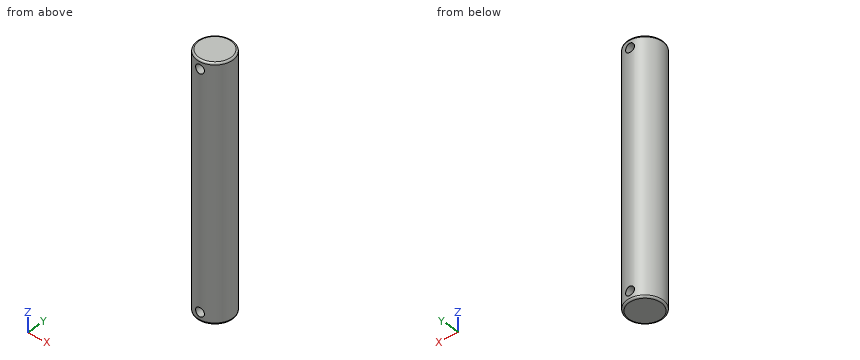
from build123d import *

# Parameters (mm, degrees)
SKETCH1_R               = 10
BOSS_EXTRUDE1_DEPTH     = 140
FILLET1_R               = 1
CUT_EXTRUDE1_DEPTH      = 140
CUT_EXTRUDE1_DEPTH_BACK = 140
SKETCH2_R               = 2.5


with BuildPart() as part:
    # Sketch1 → Boss-Extrude1 (new body)
    with BuildSketch(Plane.XY):
        Circle(SKETCH1_R)
    extrude(amount=BOSS_EXTRUDE1_DEPTH)

    # Fillet1
    fillet1_edges = [part.edges().sort_by_distance(p)[0] for p in [
        (-10, 0, 0),
        (-10, 0, 140),
    ]]
    fillet(fillet1_edges, radius=FILLET1_R)

    # Sketch2 → Cut-Extrude1 (cut, two sides: drawn at the far end of the back side and taken through both)
    with BuildSketch(Plane(origin=(0, 0, 0), x_dir=(1, 0, 0), z_dir=(0, 1, 0)).offset(-CUT_EXTRUDE1_DEPTH_BACK)):
        with Locations(Location((0, -5, 0), (0, 0, 90))):
            Circle(SKETCH2_R)
        with Locations(Location((0, -135, 0), (0, 0, 90))):
            Circle(SKETCH2_R)
    extrude(amount=CUT_EXTRUDE1_DEPTH + CUT_EXTRUDE1_DEPTH_BACK, mode=Mode.SUBTRACT)


solid = part.part
Design review of the part built by this model. Coordinates are the model's own, in mm. Coordinates: 2 decimals unless noted, no trailing zeros. Write each loop counter-clockwise with the first axis right and the second up, starting at its lowest first coordinate (ties: lowest second). Pieces come first, ordered by that corner, then holes. Notation, with made-up numbers: (-33.5, 48) -> (-23.5, 48) arc R17 ccw to (-23.5, 72) -> close; hole circle Ø10 at (-14.75, 25). An arc over 180 degrees is marked (long way). Write each question's results on one line, items separated by ' | '. Start each with the question number.
(1) Take a section at A-A on x = 0. Write out the cut boundary in (y, z), and give its area (3 significant figures).
(2) Take a section at B-B on z = 58. Write out the cut boundary in (x, y).
(3) Take a section at C-C on y = 3.25. Give the number of separate pieces and of enclosed holes in the cut face, and give its area (3 significant figures).
(4) Clearance check with flat-ended pins moving along their axes: P1, Ø1.5, axis at x = 8, z = 107.5, coming from the -Y side; P2, Ø4.5, axis at x = 0, z = 5, coming from the -Y side; P3, Ø6, axis at x = 7.5, z = 84.5, coming from the +Y side. State where each tip first meets the part, or that it passes through.
(5) Take a section at D-D on z = 5. Write out the cut boundary in (x, y).
(6) For line 1 along Z through (x, y) = (-1.75, -3.25); line 2 along Z through (x, y) = (0.5, -7); line 3 along X through (y, z) = (3.5, 5), list the stretches that pass through material, from the lowest coordinate up. Write a range as from..to.
Results found:
1) outline: (-10, 1) arc R1 ccw to (-9, 0) -> (9, 0) arc R1 ccw to (10, 1) -> (10, 2.5) -> (-10, 2.5) -> close; (-10, 7.5) -> (10, 7.5) -> (10, 132.5) -> (-10, 132.5) -> close; (-10, 137.5) -> (10, 137.5) -> (10, 139) arc R1 ccw to (9, 140) -> (-9, 140) arc R1 ccw to (-10, 139) -> close | area: 2,600 mm2
2) outline: circle Ø20 at (0, 0)
3) separate pieces: 1 | enclosed holes: 2 | area: 2,610 mm2
4) P1: stops at y = -6.89 | P2: passes through | P3: stops at y = 8.93
5) outline: (-2.5, -9.68) -> (-2.5, 9.68) arc R10 ccw to start; (2.5, -9.68) arc R10 ccw to (2.5, 9.68) -> close
6) line 1: z = 0..3.21, 6.79..133.21, 136.79..140 | line 2: z = 0..2.55, 7.45..132.55, 137.45..140 | line 3: x = -9.37..-2.5, 2.5..9.37
